Study the drawing (mm; zero at the part's minimum x, y, z) and answer. A direction names the side the tool comes from. Round coordinates to 2 decimals unless told otherwise and drop trailing zeros. Loops run counter-clockwise (first coordinate to the right, second up) from the corner with the lowest first, then second, coordinate; pieces in that order, holes last. Notation, with made-up numbers: (-26, 77) -> (10, 77) arc R22 ccw to (10, 98) -> close; hole circle Ø9 at (30.25, 80.25). An arc over 180 degrees is marked (long way). Use one line per item in the form item = value.
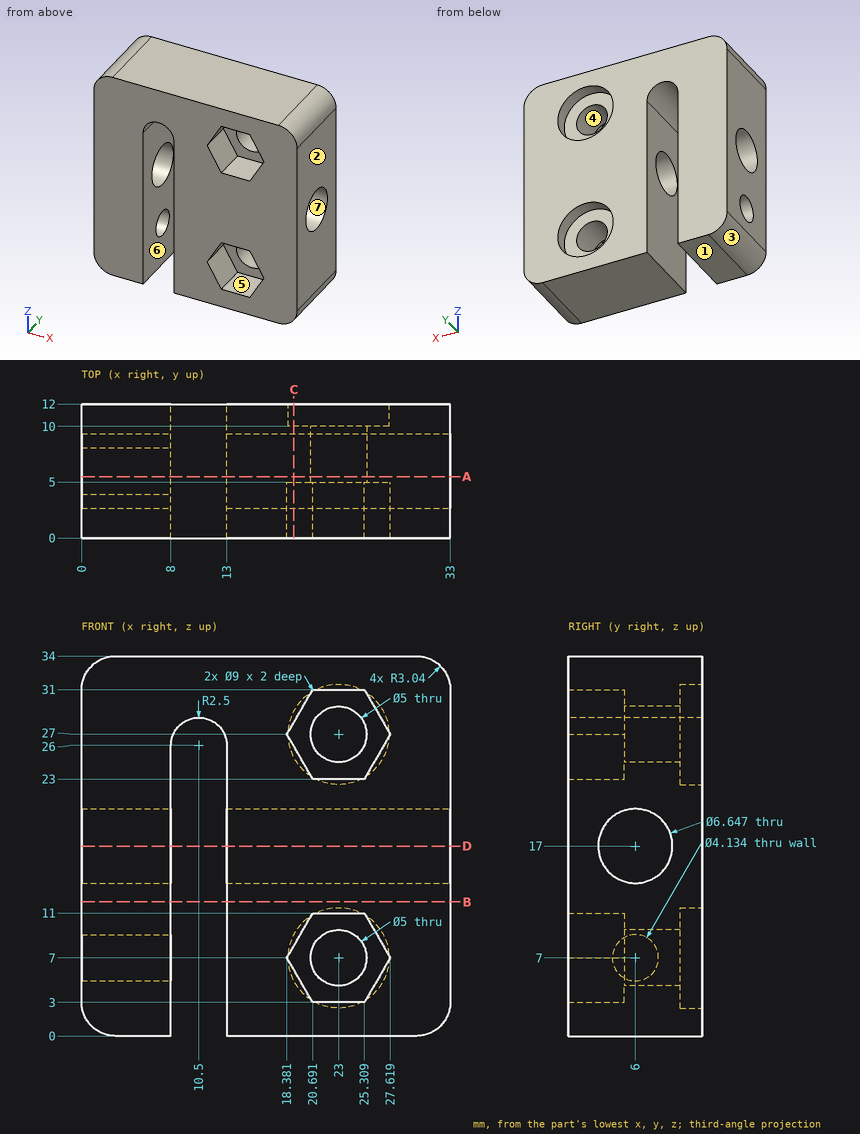
(1) Find section C-C, the plane x = 19. Write down the section's boundary in (y, z), then the cut area to 3 significant figures.
Completed:
outline = (0, 0) -> (12, 0) -> (12, 4.94) -> (10, 4.94) -> (10, 9.06) -> (12, 9.06) -> (12, 24.94) -> (10, 24.94) -> (10, 29.06) -> (12, 29.06) -> (12, 34) -> (0, 34) -> (0, 28.07) -> (5, 28.07) -> (5, 25.93) -> (0, 25.93) -> (0, 8.07) -> (5, 8.07) -> (5, 5.93) -> (0, 5.93) -> close; hole circle Ø6.65 at (6, 17)
area = 335 mm2
(2) Consider L1, parallel to Z at x = 23, y = 11.25; L2, parallel to Z at x = 4.5, y = 4.5 (1 decimal); L3, parallel to X at y = 8.5, z = 6. Determine where each line is inside the solid, lowest interval first.
Completed:
L1 = 0 to 2.5, 11.5 to 22.5, 31.5 to 34
L2 = 0 to 5.6, 8.4 to 14, 20 to 34
L3 = 0 to 8, 13 to 20.71, 25.29 to 33
(3) Find section B-B, the plane z = 12. Write down the section's boundary in (x, y).
Completed:
outline = (0, 0) -> (8, 0) -> (8, 12) -> (0, 12) -> close; (13, 0) -> (33, 0) -> (33, 12) -> (13, 12) -> close
(4) Find section D-D, the plane z = 17. Write down the section's boundary in (x, y), then the cut area to 3 significant figures.
Completed:
outline = (0, 0) -> (8, 0) -> (8, 2.68) -> (0, 2.68) -> close; (0, 9.32) -> (8, 9.32) -> (8, 12) -> (0, 12) -> close; (13, 0) -> (33, 0) -> (33, 2.68) -> (13, 2.68) -> close; (13, 9.32) -> (33, 9.32) -> (33, 12) -> (13, 12) -> close
area = 150 mm2
(5) For a pull along X with two mould halves and no side action, classify the marked faces 1, 2, 3 and 4 as +X half, -X half, draft (parallel to the pull), parting line (faces both ways), or undercut.
Completed:
face_1 = draft
face_2 = +X half
face_3 = -X half
face_4 = undercut
(6) Given P1, Ø5, axis at y = 6, z = 7, coming from the -X side; P2, Ø5.5, axis at x = 23, z = 27, coming from the -Y side; P3, Ø2.5, axis at x = 22.5, z = 28, coming from the +Y side; P4, Ø7, axis at x = 23, z = 7, coming from the +Y side, each flat-ended and moving along its own axis, determine where each tip first touches the part or whether it passes through.
Completed:
P1 = 0
P2 = 5
P3 = through
P4 = 10
(7) For the marked faces 5, 6 and 7, determine the directions among +Z, -Z, +X, -X, +Y, -Y from which every point of the face is accessible in a straight line to the end or side of a thin tool.
Completed:
face_5 = -Y
face_6 = -Z, +Y, -Y
face_7 = +X, -X
(8) Find section A-A, the plane y = 5.5. Write down the section's boundary in (x, z) (1 decimal).
Completed:
outline = (0, 3) arc R3 ccw to (3, 0) -> (8, 0) -> (8, 5) -> (0, 5) -> close; (0, 9) -> (8, 9) -> (8, 13.7) -> (0, 13.7) -> close; (0, 20.3) -> (8, 20.3) -> (8, 26) arc R2.5 cw to (13, 26) -> (13, 20.3) -> (33, 20.3) -> (33, 31) arc R3 ccw to (30, 34) -> (3, 34) arc R3 ccw to (0, 31) -> close; (13, 0) -> (30, 0) arc R3 ccw to (33, 3) -> (33, 13.7) -> (13, 13.7) -> close; hole circle Ø5 at (23, 7); hole circle Ø5 at (23, 27)
